For this review, take the finished solid that the model builds, in its own axes (mm). A direction names the side the tool comes from. Round coordinates to 2 decimals unless told otherwise and drop trailing zeros. Write each loop counter-clockwise with the first axis right and the second up, starting at its lowest first coordinate (ties: lowest second). Pieces come first, ordered by that corner, then holes. Notation, with made-up numbers: M 61.25,-19 L 83.25,-19 A30 ccw 83.25,20 Z; hole C 61,0.5 d1. An arc over 180 degrees is marked long. One line per question, with ' | ' between items.
Autodesk Inventor part; units mm, degrees
ref_plane "YZ Plane" through (0, 0, 0) normal (1, 0, 0) x (0, 1, 0)
ref_plane "XZ Plane" through (0, 0, 0) normal (0, 1, 0) x (-1, 0, 0)
ref_plane "XY Plane" through (0, 0, 0) normal (0, 0, 1) x (1, 0, 0)
sketch "Sketch1" plane through (0, 0, 0) normal (0, 0, 1) x (1, 0, 0)
  circle A0 centre (0, 0) radius 6
  circle A1 centre (0, 0) radius 17.5
  dimension "d0" = 12
  dimension "d1" = 35
extrude "Extrusion1" add sketch "Sketch1" along normal blind 10
sketch "Sketch4" plane through (0, 0, 0) normal (0, 0, -1) x (-1, 0, 0)
  circle A0 centre (0, 0) radius 13 construction
  point P0 (0, -13)
  point P1 (0, 13)
  dimension "d7" = 26
hole "Hole1" at (0, -13, 0) at (0, 13, 0) direction (0, 0, 1) diameter 5 end through all
sketch "Sketch5" plane through (0, 0, 0) normal (0, 0, -1) x (-1, 0, 0)
  circle A0 centre (0, 0) radius 8.15
  dimension "d15" = 16.3
extrude "Extrusion3" cut sketch "Sketch5" against normal blind 5
sketch "Sketch6" plane through (0, 0, 10) normal (0, 0, 1) x (1, 0, 0)
  arc A0 (25.0591, 16.1) -> (25.0591, -16.1) centre (25.0591, 0) ccw
  arc A1 (25.0591, 17.1) -> (25.0591, -17.1) centre (25.0591, 0) ccw
  circle A2 centre (0, 0) radius 17.5
  point P0 (12.8057, 11.9274)
  point P1 (12.8057, -11.9274)
  point P2 (13.4681, 11.174)
  point P3 (13.4681, -11.174)
  dimension "d22" = 1
extrude "Extrusion4" cut sketch "Sketch6" against normal through all contours A2 A0
fillet "Fillet1" radius 2 2 edges at (13.4681, -11.174, 5) (13.4681, 11.174, 5)
properties part number "Suport_Rulment" material "ABS Plastic"
Item 1: Take a section at D-D (x = -7). Write out the cut boundary in (y, z), then the cut area to 3 significant figures.
Results:
outline: M -16.04,0 L -4.17,0 L -4.17,5 L 4.17,5 L 4.17,0 L 16.04,0 L 16.04,10 L -16.04,10 Z | area: 279 mm2
Item 2: Take a section at A-A (x = 0). Write out the cut boundary in (y, z), then the cut area to 4 significant figures.
Results:
outline: M -17.5,0 L -15.5,0 L -15.5,10 L -17.5,10 Z; M -10.5,0 L -8.15,0 L -8.15,5 L -6,5 L -6,10 L -10.5,10 Z; M 6,5 L 8.15,5 L 8.15,0 L 10.5,0 L 10.5,10 L 6,10 Z; M 15.5,0 L 17.5,0 L 17.5,10 L 15.5,10 Z | area: 108.5 mm2
Item 3: Mouldability with a two-part tool opening along X and no side actions: class faces 1 (the face through (-6, 4, 10)), 2 (the face through (-17.49, -0.57, 4.93)), 3 (the face through (-6, 0, 7)) as +X half, -X half, draft (parallel to the pull), parting line (faces both ways), or undercut.
Results:
face 1: draft | face 2: parting line | face 3: undercut
Item 4: Insertion check: pin 1 Ø1.5 at (x, z) = (-5, 7.5) entering from +Y; pin 2 Ø1 at (x, z) = (5.5, 7) entering from -Y; pin 3 Ø13 at (x, y) = (0, 0) entering from -Z. Each pin has a flat end and moves straight along its axis. Give the tip position at first contact, or say it passes through.
Results:
pin 1: y = 16.98 | pin 2: y = -16.77 | pin 3: z = 5
Item 5: Take a section at B-B (y = 0). Write out the cut boundary in (x, z).
Results:
outline: M -17.5,0 L -8.15,0 L -8.15,5 L -6,5 L -6,10 L -17.5,10 Z; M 6,5 L 8.15,5 L 8.15,0 L 8.96,0 L 8.96,10 L 6,10 Z
Item 6: Take a section at C-C (z = 2.5). State how many separate pieces and enclosed holes the cut face has, then the cut area to 3 significant figures.
Results:
separate pieces: 1 | enclosed holes: 3 | area: 582 mm2
Item 7: Machinability: for faces 4 (the face through (-9, 0, 0)), 5 (the face through (6.468, -4.959, 2.465)), which of the approach directions +Z, -Z, +X, -X, +Y, -Y give a long, thin tool a straight path to every point of the face, cutting with its end or side? Answer none if there is none.
Results:
face 4: -Z, +X, -X, +Y, -Y | face 5: -Z
Item 8: To check wall thickness, follow line 1 along Y through (x, z) = (0, 5.75); line 2 along Y through (x, z) = (0, 2); line 3 along Y through (x, z) = (5, 9.5). State the ranges of each line that lie inside material, in increasing order. Write a range as from..to.
Results:
line 1: -17.5..-15.5, -10.5..-6, 6..10.5, 15.5..17.5 | line 2: -17.5..-15.5, -10.5..-8.15, 8.15..10.5, 15.5..17.5 | line 3: -16.77..-3.32, 3.32..16.77
